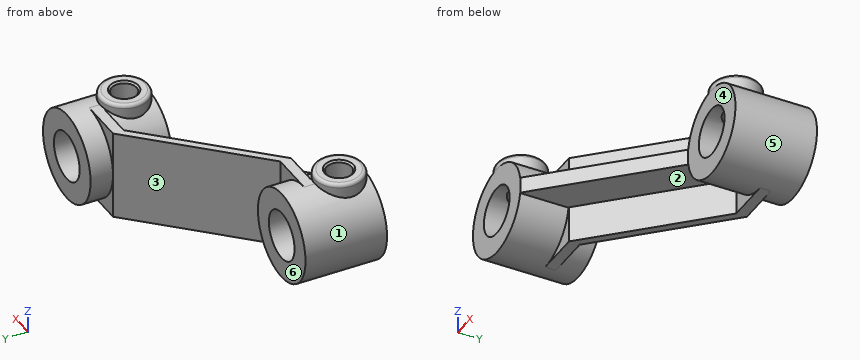
```python
from build123d import *

# Parameters (mm, degrees)
BOSS_EXTRUDE1_START     = 61.5
SKETCH2_R               = 25
SKETCH2_R_2             = 13.5
BOSS_EXTRUDE1_DEPTH     = 45.5
SKETCH2_3_R             = 25
SKETCH2_3_R_2           = 13.5
BOSS_EXTRUDE2_DEPTH     = 45.5
BOSS_EXTRUDE3_DEPTH     = 25
BOSS_EXTRUDE5_REACH     = 205.566
BOSS_EXTRUDE5_START     = 29.5
SKETCH4_R               = 13.5
RIB1_START              = -4.5
RIB1_DEPTH              = 9
FILLET1_R               = 2
CUT_EXTRUDE3_DEPTH      = 175.769133569
CUT_EXTRUDE3_DEPTH_BACK = 52.5
SKETCH10_R              = 13.5


with BuildPart() as part:
    # Sketch2 → Boss-Extrude1 (new body)
    with BuildSketch(Plane(origin=(0, 0, 0), x_dir=(1, 0, 0), z_dir=(0, 1, 0)).offset(BOSS_EXTRUDE1_START)):
        with Locations(Location((110, 0, 0), (0, 0, 270))):
            Circle(SKETCH2_R)
        with Locations(Location((110, 0, 0), (0, 0, 270))):
            Circle(SKETCH2_R_2, mode=Mode.SUBTRACT)
    extrude(amount=BOSS_EXTRUDE1_DEPTH)



with BuildPart() as body_2:
    # Sketch2<3> → Boss-Extrude2 (new body)
    with BuildSketch(Plane(origin=(0, 0, 0), x_dir=(1, 0, 0), z_dir=(0, 1, 0))):
        with Locations(Location((0, 0, 0), (0, 0, 270))):
            Circle(SKETCH2_3_R)
        with Locations(Location((0, 0, 0), (0, 0, 270))):
            Circle(SKETCH2_3_R_2, mode=Mode.SUBTRACT)
    extrude(amount=BOSS_EXTRUDE2_DEPTH)


with BuildPart() as part_1:
    add(part.part)

    add(body_2.part)  # Boss-Extrude3 merges body 2
    # Sketch3 → Boss-Extrude3 (add, symmetric)
    with BuildSketch(Plane.XY):
        Polygon((0, 27), (25, 27), (85, 88.5), (110, 88.5), (110, 94.5), (85, 94.5), (25, 33), (0, 33), align=None)
    extrude(amount=BOSS_EXTRUDE3_DEPTH, both=True)

    # Sketch4 → Boss-Extrude5 (add, up to next)
    with BuildSketch(Plane.XY.offset(BOSS_EXTRUDE5_START), mode=Mode.PRIVATE) as boss_extrude5_sk1:
        with Locations((0, 13.5)):
            Circle(SKETCH4_R)
    boss_extrude5_tool1 = extrude(boss_extrude5_sk1.sketch, amount=-BOSS_EXTRUDE5_REACH, mode=Mode.PRIVATE) - part_1.part
    # Sketch4 → Boss-Extrude5 (add, up to next)
    with BuildSketch(Plane.XY.offset(BOSS_EXTRUDE5_START), mode=Mode.PRIVATE) as boss_extrude5_sk2:
        with Locations((110, 75)):
            Circle(SKETCH4_R)
    boss_extrude5_tool2 = extrude(boss_extrude5_sk2.sketch, amount=-BOSS_EXTRUDE5_REACH, mode=Mode.PRIVATE) - part_1.part
    add(boss_extrude5_tool1.solids().sort_by_distance((0, 13.5, 29.5))[0])
    add(boss_extrude5_tool2.solids().sort_by_distance((110, 75, 29.5))[0])

    # Rib1: read off the stored shape, not the designer's step
    # Rib1 outline → Rib1 (add)
    with BuildSketch(Plane.XY.offset(RIB1_START)):
        Polygon((85, 61.5), (85.408334745, 61.5), (85.408334745, 88.5), (85, 88.5), (25, 27), (24.591665255, 27), (24.591665255, 0), (25, 0), align=None)
    extrude(amount=RIB1_DEPTH)

    # CSK for M16 SFHCS1: read off the stored shape, not the designer's step
    # CSK for M16 SFHCS1 outline → CSK for M16 SFHCS1 (revolve, cut)
    with BuildSketch(Plane(origin=(110, 75, 0), x_dir=(1, 0, 0), z_dir=(0, -1, 0))):
        Polygon((0, 11.543091406), (7, 11.543091406), (7, 28.5), (8, 29.5), (0, 29.5), align=None)
    revolve(axis=Axis((110, 75, 0), (0, 0, 1)), mode=Mode.SUBTRACT)

    # CSK for M16 SFHCS1 2 outline → CSK for M16 SFHCS1 2 (revolve, cut)
    with BuildSketch(Plane.XZ.offset(-13.5)):
        Polygon((0, 11.543091406), (7, 11.543091406), (7, 28.5), (8, 29.5), (0, 29.5), align=None)
    revolve(axis=Axis((0, 13.5, 0), (0, 0, 1)), mode=Mode.SUBTRACT)

    # Fillet1
    fillet1_edges = [part_1.edges().sort_by_distance(p)[0] for p in [
        (-13.5, 13.5, 29.5),
        (96.5, 75, 29.5),
    ]]
    fillet(fillet1_edges, radius=FILLET1_R)

    # Sketch10 → Cut-Extrude3 (cut, two sides: drawn at the far end of the back side and taken through both)
    with BuildSketch(Plane(origin=(0, 0, 0), x_dir=(1, 0, 0), z_dir=(0, 1, 0)).offset(-CUT_EXTRUDE3_DEPTH_BACK)):
        with Locations(Location((0, 0, 0), (0, 0, 270))):
            Circle(SKETCH10_R)
        with Locations(Location((110, 0, 0), (0, 0, 270))):
            Circle(SKETCH10_R)
    extrude(amount=CUT_EXTRUDE3_DEPTH + CUT_EXTRUDE3_DEPTH_BACK, mode=Mode.SUBTRACT)


solid = part_1.part
```
Here's how the part is built. I have some questions about the finished solid (model axes, mm). Face numbers are marked on the shaded views. A direction names the side the tool comes from. Round coordinates to 2 decimals unless told otherwise and drop trailing zeros. Order: outer loops, then holes, each group sorted by start corner. A loop starts at its lowest first (then second) coordinate and runs counter-clockwise, first axis right, second up. Notation, with made-up numbers: (-37.75, 4.25) -> (13.25, 4.25) arc R33 ccw to (13.25, 41.25) -> close; hole circle Ø7 at (-19, 7). An arc over 180 degrees is marked (long way). Use a Markdown table: item, result. Add a question column.
(1) For pin 1 Ø20 at (x, y) = (53.5, 46.5) entering from +Z; pin 2 Ø10.5 at (x, z) = (7.5, 17) entering from -Y; pin 3 Ø6 at (x, z) = (94.5, 10) entering from -Y; pin 4 Ø12 at (x, z) = (40.5, 5.5) entering from -Y, each with a flat end and sliding along its axis, tell me the tip position at first contact or that it passes through.
(2) Suppose I cut it at C-C, the plane x = 106.5. Count the separate pieces of the cut face and the enclosed holes in it, and give its area (3 significant figures).
(3) Suppose I cut it at A-A, the plane x = 41. Please give me the cut outline in (y, z), and give its area (3 significant figures).
(4) For the marked faces 1, 2, 3 and 4, which set-ups out of +Z, -Z, +X, -X, +Y, -Y let a thin tool reach every point of the face, with its end or its side?
(5) I need wall thicknesses on line 1 along Z through (x, y) = (67, 63); line 2 along X through (y, z) = (11, 0); line 3 along Z through (x, y) = (40.5, 47.5). Which ranges of each line are inside material? Lowest first, please.
(6) Suppose I cut it at D-D, the plane y = 100. Please give me the cut outline in (x, z), and give its area (3 significant figures).
(7) Suppose I cut it at B-B, the plane y = 75. Please give me the cut outline in (x, z), and give its area (3 significant figures).
(8) If we mould it in two halves opening along X, with no side actions, what happens to the marked faces 5 and 6? For each: released by +X, released by -X, zero draft, split by the parting line, or undercut.
Verdict:
| question | item | result |
|---|---|---|
| 1 | pin 1 | z = 25 |
| 1 | pin 2 | y = 0 |
| 1 | pin 3 | y = 61.5 |
| 1 | pin 4 | y = 9.82 |
| 2 | separate pieces | 3 |
| 2 | enclosed holes | 0 |
| 2 | area | 990 mm2 |
| 3 | outline | (16.4, -4.5) -> (43.4, -4.5) -> (43.4, -25) -> (49.4, -25) -> (49.4, 25) -> (43.4, 25) -> (43.4, 4.5) -> (16.4, 4.5) -> close |
| 3 | area | 543 mm2 |
| 4 | face 1 | none |
| 4 | face 2 | -Z, -Y |
| 4 | face 3 | +Z, -Z, +Y |
| 4 | face 4 | +Z, -Z, +X, -Y |
| 5 | line 1 | -4.5 to 4.5 |
| 5 | line 2 | -25 to -13.5, 13.5 to 35.73 |
| 5 | line 3 | -25 to 25 |
| 6 | outline | circle Ø50 at (110, 0); hole circle Ø27 at (110, 0) |
| 6 | area | 1,390 mm2 |
| 7 | outline | (65.98, -25) -> (71.83, -25) -> (71.83, -4.5) -> (85.41, -4.5) arc R25 ccw (long way) to (123.5, 21.04) -> (123.5, 27.5) arc R2 ccw to (121.5, 29.5) -> (118, 29.5) -> (117, 28.5) -> (117, 11.54) arc R13.5 cw (long way) to (103, 11.54) -> (103, 28.5) -> (102, 29.5) -> (98.5, 29.5) arc R2 ccw to (96.5, 27.5) -> (96.5, 21.04) arc R25 ccw to (85.41, 4.5) -> (71.83, 4.5) -> (71.83, 25) -> (65.98, 25) -> close |
| 7 | area | 1,720 mm2 |
| 8 | face 5 | undercut |
| 8 | face 6 | zero draft |
